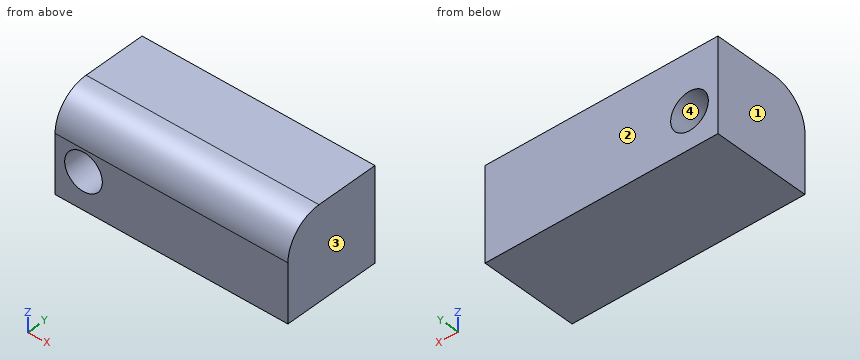
from build123d import *

# Parameters (mm, degrees)
F0_W     = 106.66725
F0_H     = 42.689698
F0_R     = 8.621606
F1_DEPTH = 44.704
F2_R     = 15.943466


with BuildPart() as f1:
    # F0 (on Front) → F1 (new body)
    with BuildSketch(Plane.XZ):
        with Locations((-18.370472, -15.969823)):
            Rectangle(F0_W, F0_H)
        with Locations((-58.666989, -20.491278)):
            Circle(F0_R, mode=Mode.SUBTRACT)
    extrude(amount=F1_DEPTH)

    # F2
    f2_edges = [f1.edges().sort_by_distance(p)[0] for p in [
        (-18.370472, -44.704, 5.375026),
    ]]
    fillet(f2_edges, radius=F2_R)


solid = f1.part
Input: part model. Units: mm. Frame: model coordinates. Face numbers are marked on the shaded views. Give positions to 0.01 mm unless a question says otherwise; leave off trailing zeros. Order: outer loops, then holes, each group sorted by start corner. A loop starts at its lowest first (then second) coordinate and runs counter-clockwise, first axis right, second up. Notation, with made-up numbers: (-1, 15.5) -> (19, 15.5) arc R22 cw to (19, 30.5) -> close; hole circle Ø7 at (-31.75, 21). An arc over 180 degrees is marked (long way). Use one line per item in the form item = value.
1) Section C-C, the plane x = 14. Return loops of the section in (y, z), and give its area (3 significant figures).
Response values:
outline = (-44.7, -37.31) -> (0, -37.31) -> (0, 5.38) -> (-28.76, 5.38) arc R15.94 ccw to (-44.7, -10.57) -> close
area = 1,850 mm^2
2) Line query: probe 1 along X at (y, z) = (-17.5, -21); probe 2 along Y at (x, z) = (-56.5, -10.5); probe 3 along Z at (x, y) = (-53.5, -24.5). Output: solid intervals per line, ascending.
Response values:
probe_1 = -71.7 to -67.27, -50.06 to 34.96
probe_2 = -44.7 to 0
probe_3 = -37.31 to -27.39, -13.59 to 5.38
3) Section A-A, the plane z = -27. Return loops of the section in (x, y), and give its area (3 significant figures).
Response values:
outline = (-71.7, -44.7) -> (-64.32, -44.7) -> (-64.32, 0) -> (-71.7, 0) -> close; (-53.01, -44.7) -> (34.96, -44.7) -> (34.96, 0) -> (-53.01, 0) -> close
area = 4,260 mm^2
4) Section D-D, the plane z = -16.5. Return loops of the section in (x, y).
Response values:
outline = (-71.7, -44.7) -> (-66.31, -44.7) -> (-66.31, 0) -> (-71.7, 0) -> close; (-51.02, -44.7) -> (34.96, -44.7) -> (34.96, 0) -> (-51.02, 0) -> close
5) Section B-B, the plane y = -41. Return loops of the section in (x, z), and give its area (3 significant figures).
Response values:
outline = (-71.7, -37.31) -> (34.96, -37.31) -> (34.96, -0.35) -> (-71.7, -0.35) -> close; hole circle Ø17.24 at (-58.67, -20.49)
area = 3,710 mm^2
6) First-contact query: pin 1 Ø1.5 at (x, z) = (22, -6) entering from -Y. Flat tip, straight axial feed; report the tip coordinate or a pass-through.
Response values:
pin_1 = -44.24
7) Mould query, pull axis X, two halves, no side actions, for the marked faces 1, 2, 3 and 4. Classes: pulls with the +X half, pulls with the -X half, needs draft (parallel to the pull), parting line crosses it, or undercut.
Response values:
face_1 = pulls with the -X half
face_2 = needs draft
face_3 = pulls with the +X half
face_4 = undercut
